```python
from build123d import *

# Parameters (mm, degrees)
SKETCH1_W           = 100.4
SKETCH1_H           = 113.4
BOSS_EXTRUDE1_DEPTH = 5
SKETCH2_W           = 90.4
SKETCH2_H           = 103.4
BOSS_EXTRUDE2_DEPTH = 5
FILLET1_R           = 5
SKETCH3_R           = 1.5
CUT_EXTRUDE1_DEPTH  = 17
SKETCH4_R           = 3
CUT_EXTRUDE2_DEPTH  = 4
SKETCH5_R           = 0.75
CUT_EXTRUDE3_DEPTH  = 19


with BuildPart() as part:
    # Sketch1 → Boss-Extrude1 (new body)
    with BuildSketch(Plane(origin=(0, 0, 0), x_dir=(1, 0, 0), z_dir=(0, 1, 0))):
        Rectangle(SKETCH1_W, SKETCH1_H)
    extrude(amount=BOSS_EXTRUDE1_DEPTH)

    # Sketch2 → Boss-Extrude2 (add)
    with BuildSketch(Plane.XZ):
        Rectangle(SKETCH2_W, SKETCH2_H)
    extrude(amount=BOSS_EXTRUDE2_DEPTH)

    # Fillet1
    fillet1_edges = [part.edges().sort_by_distance(p)[0] for p in [
        (50.2, 2.5, 56.7),
        (-50.2, 2.5, 56.7),
        (-50.2, 2.5, -56.7),
        (50.2, 2.5, -56.7),
    ]]
    fillet(fillet1_edges, radius=FILLET1_R)

    # Sketch3 → Cut-Extrude1 (cut)
    with BuildSketch(Plane(origin=(0, 5, 0), x_dir=(1, 0, 0), z_dir=(0, 1, 0))):
        with Locations((-35.2, 36.65)):
            Circle(SKETCH3_R)
        with Locations((-35.2, -36.65)):
            Circle(SKETCH3_R)
        with Locations((35.2, 36.65)):
            Circle(SKETCH3_R)
        with Locations((35.2, -36.65)):
            Circle(SKETCH3_R)
    extrude(amount=-CUT_EXTRUDE1_DEPTH, mode=Mode.SUBTRACT)

    # Sketch4 → Cut-Extrude2 (cut)
    with BuildSketch(Plane(origin=(0, 5, 0), x_dir=(1, 0, 0), z_dir=(0, 1, 0))):
        with Locations((-35.2, 36.65)):
            Circle(SKETCH4_R)
        with Locations((-35.2, -36.65)):
            Circle(SKETCH4_R)
        with Locations((35.2, 36.65)):
            Circle(SKETCH4_R)
        with Locations((35.2, -36.65)):
            Circle(SKETCH4_R)
    extrude(amount=-CUT_EXTRUDE2_DEPTH, mode=Mode.SUBTRACT)

    # Sketch5 → Cut-Extrude3 (cut)
    with BuildSketch(Plane(origin=(0, 5, 0), x_dir=(1, 0, 0), z_dir=(0, 1, 0))):
        with Locations((-24.945666125, 42.299983599)):
            Circle(SKETCH5_R)
        with Locations((-25, -47.7)):
            Circle(SKETCH5_R)
        with Locations((25.054333875, 42.299983599)):
            Circle(SKETCH5_R)
        with Locations((25, -47.7)):
            Circle(SKETCH5_R)
    extrude(amount=-CUT_EXTRUDE3_DEPTH, mode=Mode.SUBTRACT)


solid = part.part
```
Geometry check sheet. Reference: the model listing, model coordinates, mm. A direction names the side the tool comes from. Round coordinates to 2 decimals unless told otherwise and drop trailing zeros. Order: outer loops, then holes, each group sorted by start corner. A loop starts at its lowest first (then second) coordinate and runs counter-clockwise, first axis right, second up. Notation, with made-up numbers: (-27.5, -37) - (29.5, -37) arc R27 ccw to (29.5, -6) - close; hole circle Ø8 at (-9.5, 8.5). An arc over 180 degrees is marked (long way). Use a Markdown table: item, result. Add a question column.
1) Set-up check for faces 5 (the flat face through (36, 1, 35)), 6 (the cylindrical face through (34.01, -1.96, 37.56)), 7 (the flat face through (-45.2, -2, -1)): record each of +Z, -Z, +X, -X, +Y, -Y from which the full face is reachable in a straight line by a thin tool's end or side.
2) Section check A-A (x = 35.2). Record the cut outline in (y, z).
3) Gauge pin test, flat ends, axial feed: P1, Ø2.5, axis at x = 15, y = -1.5, coming from the +Z side; P2, Ø5.5, axis at x = -35.2, z = 36.65, coming from the +Y side; P3, Ø2, axis at x = 25, z = 47.7, coming from the -Y side; P4, Ø3, axis at y = -2, z = -2.5, coming from the +X side. Record the tip position at first contact, or that the pin passes through.
4) Section check C-C (z = 0). Record the cut outline in (x, y), then the cut area to 3 significant figures.
5) Thickness scan on line 1 along X through (y, z) = (-0.5, 47.7); line 2 along Z through (x, y) = (35.2, -2.25); line 3 along X through (y, z) = (4.2, -36.65). Record the ranges inside material, lowest first.
6) Section check B-B (z = 36.65). Record the cut outline in (x, y), then the cut area to 3 significant figures.
7) Section check D-D (x = -0.5). Record the cut outline in (y, z).
8) Mould release check, pull along Z, two halves, no side actions. Record for faces 1 (the flat face through (34, 1, -38)), 2 (the flat face through (-1, -2, 51.7)), 3 (the flat face through (-1, 5, -1)), 4 (the cylindrical face through (32.819, 3.028, 38.475)): released by +Z, released by -Z, zero draft, split by the parting line, or undercut.
Established:
| question | item | result |
|---|---|---|
| 1 | face 5 | +Y |
| 1 | face 6 | +Y, -Y |
| 1 | face 7 | +Z, -Z, -X, -Y |
| 2 | outline | (-5, -51.7) - (0, -51.7) - (0, -56.7) - (5, -56.7) - (5, -39.65) - (1, -39.65) - (1, -38.15) - (-5, -38.15) - close; (-5, -35.15) - (1, -35.15) - (1, -33.65) - (5, -33.65) - (5, 33.65) - (1, 33.65) - (1, 35.15) - (-5, 35.15) - close; (-5, 38.15) - (1, 38.15) - (1, 39.65) - (5, 39.65) - (5, 56.7) - (0, 56.7) - (0, 51.7) - (-5, 51.7) - close |
| 3 | P1 | z = 51.7 |
| 3 | P2 | y = 1 |
| 3 | P3 | y = -5 |
| 3 | P4 | x = 45.2 |
| 4 | outline | (-50.2, 0) - (-45.2, 0) - (-45.2, -5) - (45.2, -5) - (45.2, 0) - (50.2, 0) - (50.2, 5) - (-50.2, 5) - close |
| 4 | area | 954 mm2 |
| 5 | line 1 | -45.2 to -25.75, -24.25 to 24.25, 25.75 to 45.2 |
| 5 | line 2 | -51.7 to -38.15, -35.15 to 35.15, 38.15 to 51.7 |
| 5 | line 3 | -50.2 to -38.2, -32.2 to 32.2, 38.2 to 50.2 |
| 6 | outline | (-50.2, 0) - (-45.2, 0) - (-45.2, -5) - (-36.7, -5) - (-36.7, 1) - (-38.2, 1) - (-38.2, 5) - (-50.2, 5) - close; (-33.7, -5) - (33.7, -5) - (33.7, 1) - (32.2, 1) - (32.2, 5) - (-32.2, 5) - (-32.2, 1) - (-33.7, 1) - close; (36.7, -5) - (45.2, -5) - (45.2, 0) - (50.2, 0) - (50.2, 5) - (38.2, 5) - (38.2, 1) - (36.7, 1) - close |
| 6 | area | 870 mm2 |
| 7 | outline | (-5, -51.7) - (0, -51.7) - (0, -56.7) - (5, -56.7) - (5, 56.7) - (0, 56.7) - (0, 51.7) - (-5, 51.7) - close |
| 8 | face 1 | undercut |
| 8 | face 2 | released by +Z |
| 8 | face 3 | zero draft |
| 8 | face 4 | undercut |
